```python
from build123d import *

# Parameters (mm, degrees)
SKETCH1_R           = 1.5367
BOSS_EXTRUDE1_DEPTH = 1.6
FILLET1_R           = 2.54
SKETCH3_R           = 1.5367
CUT_EXTRUDE1_DEPTH  = 2.6


with BuildPart() as part:
    # Sketch1 → Boss-Extrude1 (new body)
    with BuildSketch(Plane.XY):
        with BuildLine():
            Line((7.903015948, 75.005885785), (7.903015948, 68.549399108))
            ThreePointArc((7.903015948, 68.549399108), (9.403015948, 64.505885785), (7.903015948, 60.462372462))
            Line((7.903015948, 60.462372462), (7.903015948, 45.943399108))
            ThreePointArc((7.903015948, 45.943399108), (9.403015948, 41.899885785), (7.903015948, 37.856372462))
            Line((7.903015948, 37.856372462), (7.903015948, 23.337399108))
            ThreePointArc((7.903015948, 23.337399108), (9.403015948, 19.293885785), (7.903015948, 15.250372462))
            Line((7.903015948, 15.250372462), (7.903015948, 0.731399108))
            ThreePointArc((7.903015948, 0.731399108), (9.403015948, -3.312114215), (7.903015948, -7.355627538))
            Line((7.903015948, -7.355627538), (7.903015948, -13.812114215))
            Line((7.903015948, -13.812114215), (7.903015948, -18.812254411))
            Line((7.903015948, -18.812254411), (22.633015952, -18.812254411))
            Line((22.633015952, -18.812254411), (22.633015952, -13.812114215))
            Line((22.633015952, -13.812114215), (22.633015952, -7.355627538))
            ThreePointArc((22.633015952, -7.355627538), (21.133015952, -3.312114215), (22.633015952, 0.731399108))
            Line((22.633015952, 0.731399108), (22.633015952, 15.250372462))
            ThreePointArc((22.633015952, 15.250372462), (21.133015952, 19.293885785), (22.633015952, 23.337399108))
            Line((22.633015952, 23.337399108), (22.633015952, 37.856372462))
            ThreePointArc((22.633015952, 37.856372462), (21.133015952, 41.899885785), (22.633015952, 45.943399108))
            Line((22.633015952, 45.943399108), (22.633015952, 60.462372462))
            ThreePointArc((22.633015952, 60.462372462), (21.133015952, 64.505885785), (22.633015952, 68.549399108))
            Line((22.633015952, 68.549399108), (22.633015952, 75.005885785))
            Line((22.633015952, 75.005885785), (22.633015952, 80.006025981))
            Line((22.633015952, 80.006025981), (7.903015948, 80.006025981))
            Line((7.903015948, 80.006025981), (7.903015948, 75.005885785))
        make_face()
        with Locations((15.26801595, 74.583125981)):
            Circle(SKETCH1_R, mode=Mode.SUBTRACT)
        with Locations((15.26801595, -13.389354411)):
            Circle(SKETCH1_R, mode=Mode.SUBTRACT)
    extrude(amount=BOSS_EXTRUDE1_DEPTH)

    # Fillet1
    fillet1_edges = [part.edges().sort_by_distance(p)[0] for p in [
        (7.903015948, 80.006025981, 0.8),
        (22.633015952, 80.006025981, 0.8),
        (22.633015952, 68.549399108, 0.8),
        (22.633015952, 60.462372462, 0.8),
        (22.633015952, 45.943399108, 0.8),
        (22.633015952, 37.856372462, 0.8),
        (22.633015952, 23.337399108, 0.8),
        (22.633015952, 15.250372462, 0.8),
        (22.633015952, 0.731399108, 0.8),
        (22.633015952, -7.355627538, 0.8),
        (22.633015952, -18.812254411, 0.8),
        (7.903015948, -18.812254411, 0.8),
        (7.903015948, -7.355627538, 0.8),
        (7.903015948, 0.731399108, 0.8),
        (7.903015948, 15.250372462, 0.8),
        (7.903015948, 23.337399108, 0.8),
        (7.903015948, 37.856372462, 0.8),
        (7.903015948, 45.943399108, 0.8),
        (7.903015948, 60.462372462, 0.8),
        (7.903015948, 68.549399108, 0.8),
    ]]
    fillet(fillet1_edges, radius=FILLET1_R)

    # Sketch3 → Cut-Extrude1 (cut, through all)
    with BuildSketch(Plane.XY.offset(1.6)):
        with Locations((15.26801595, 30.596885785)):
            Circle(SKETCH3_R)
    extrude(amount=-CUT_EXTRUDE1_DEPTH, mode=Mode.SUBTRACT)


solid = part.part
```
Input: part model. Units: mm. Frame: model coordinates. Give positions to 0.01 mm unless a question says otherwise; leave off trailing zeros. Order: outer loops, then holes, each group sorted by start corner. A loop starts at its lowest first (then second) coordinate and runs counter-clockwise, first axis right, second up. Notation, with made-up numbers: (83.5, 23) - (123.5, 23) arc R16 ccw to (123.5, 52) - close; hole circle Ø1 at (50, -28). An arc over 180 degrees is marked (long way). Use a Markdown table: item, result.
(1) Section query C-C (y = 40). Output: boundary loops of the cut face in (x, z), then the cut area to 3 significant figures.
Computed values:
| item | result |
|---|---|
| outline | (9.1, 0) - (21.43, 0) - (21.43, 1.6) - (9.1, 1.6) - close |
| area | 19.7 mm2 |
(2) Section query A-A (y = 63.5). Output: boundary loops of the cut face in (x, z).
Computed values:
| item | result |
|---|---|
| outline | (9.32, 0) - (21.22, 0) - (21.22, 1.6) - (9.32, 1.6) - close |
(3) Line query: line 1 (Y direction, x = 15, z = 0.25); line 2 (Y direction, x = 14, z = 0.2); line 3 (X direction, y = 29.5, z = 0.95). Output: solid intervals per line, ascending. Write a range as from..to.
Computed values:
| item | result |
|---|---|
| line 1 | y = -18.81..-14.9, -11.88..29.08, 32.11..73.07, 76.1..80.01 |
| line 2 | y = -18.81..-14.26, -12.52..29.73, 31.46..73.72, 75.45..80.01 |
| line 3 | x = 7.9..14.19, 16.34..22.63 |
(4) Section query B-B (z = 1.2). State how many separate pieces and enclosed holes the cut face has, then the cut area to 3 significant figures.
Computed values:
| item | result |
|---|---|
| separate pieces | 1 |
| enclosed holes | 3 |
| area | 1,360 mm2 |
(5) Draft query along X for faces 1 (the cylindrical face through (15.98, -14.75, 0.79)), 2 (the flat face through (22.633, -12, 1)), 3 (the cylindrical face through (9.403, -3.261, 0.789)), 4 (the flat face through (15, -18.812, 1)). Return one class per face: released by +X, released by -X, zero draft, split by the parting line, or undercut.
Computed values:
| item | result |
|---|---|
| face 1 | undercut |
| face 2 | released by +X |
| face 3 | released by -X |
| face 4 | zero draft |
